Verification items for the finished model (mm, model axes). A direction names the side the tool comes from. Coordinates: 2 decimals unless noted, no trailing zeros. Loops run counter-clockwise (first coordinate to the right, second up) from the corner with the lowest first, then second, coordinate; pieces in that order, holes last.
Q1. Access from +Z, -Z, +X, -X, +Y, -Y to the whole of each face (thin tool, end or side, straight path). Record for faces 4 (the face through (12, 30, -25)), 5 (the face through (82, 42.5, -25)), 6 (the face through (50, 10, -25)), 7 (the face through (11.198, 17.325, -34.915)).
Q2. Sectioned sample at D-D (z = -25). Enter the section's corners in (x, y).
Q3. Sectioned sample at A-A (x = 12.5). Enter the section's corners in (y, z), then the cut area to 3 significant figures.
Q4. Sectioned sample at B-B (y = 6). Enter the section's corners in (x, z), then the cut area to 3 significant figures.
Q5. Go/stop test with flat-tipped pins: P1, Ø1.5, axis at y = 23.5, z = -19.5, coming from the -X side; P2, Ø6, axis at y = 27.5, z = -30.5, coming from the -X side; P3, Ø1.5, axis at x = 10, y = 23, coming from the -Z side. Record where each tip stops, or that it passes through.
Q6. Sectioned sample at C-C (y = 17.5). Enter the section's corners in (x, z).
Q7. Material ranges on probe 1 along X at (y, z) = (6, -21.5); probe 2 along Y at (x, z) = (19.5, -21); probe 3 along Y at (x, z) = (29.5, -5), recorded low to high.
Q8. Mould release check, pull along X, two halves, no side actions. Record for faces 1 (the face through (100, 2, -25)), 2 (the face through (49, 2, -50)), 3 (the face through (38, 5, -25)): +X half, -X half, draft (parallel to the pull), parting line (faces both ways), or undercut.
```python
from build123d import *

# Parameters (mm, degrees)
SKETCH1_W           = 100
SKETCH1_H           = 50
BOSS_EXTRUDE1_DEPTH = 5
SKETCH3_R           = 10
BOSS_EXTRUDE2_DEPTH = 25
SKETCH4_R           = 11.25
BOSS_EXTRUDE3_DEPTH = 5
SKETCH5_R           = 12.5
BOSS_EXTRUDE4_DEPTH = 37.5


with BuildPart() as part:
    # Sketch1 → Boss-Extrude1 (new body)
    with BuildSketch(Plane(origin=(0, 0, 0), x_dir=(1, 0, 0), z_dir=(0, 1, 0))):
        with Locations((50, 25)):
            Rectangle(SKETCH1_W, SKETCH1_H)
    extrude(amount=BOSS_EXTRUDE1_DEPTH)

    # Sketch3 → Boss-Extrude2 (add)
    with BuildSketch(Plane(origin=(0, 5, 0), x_dir=(1, 0, 0), z_dir=(0, 1, 0))):
        with Locations((12.5, 25)):
            Circle(SKETCH3_R)
    extrude(amount=BOSS_EXTRUDE2_DEPTH)

    # Sketch4 → Boss-Extrude3 (add)
    with BuildSketch(Plane(origin=(0, 5, 0), x_dir=(1, 0, 0), z_dir=(0, 1, 0))):
        with Locations((50, 25)):
            Circle(SKETCH4_R)
    extrude(amount=BOSS_EXTRUDE3_DEPTH)

    # Sketch5 → Boss-Extrude4 (add)
    with BuildSketch(Plane(origin=(0, 5, 0), x_dir=(1, 0, 0), z_dir=(0, 1, 0))):
        with Locations((82.5, 25)):
            Circle(SKETCH5_R)
    extrude(amount=BOSS_EXTRUDE4_DEPTH)


solid = part.part
```
Geometry check:
1. face 4: +Z, -Z, -X, +Y
1. face 5: +Z, -Z, +X, -X, +Y
1. face 6: +Z, -Z, +Y
1. face 7: +Y
2. outline: (0, 0) - (100, 0) - (100, 5) - (95, 5) - (95, 42.5) - (70, 42.5) - (70, 5) - (61.25, 5) - (61.25, 10) - (38.75, 10) - (38.75, 5) - (22.5, 5) - (22.5, 30) - (2.5, 30) - (2.5, 5) - (0, 5) - close
3. outline: (0, -50) - (5, -50) - (5, -35) - (30, -35) - (30, -15) - (5, -15) - (5, 0) - (0, 0) - close
3. area: 750 mm2
4. outline: circle Ø20 at (12.5, -25); circle Ø22.5 at (50, -25); circle Ø25 at (82.5, -25)
4. area: 1,200 mm2
5. P1: stops at x = 3.7
5. P2: stops at x = 2.82
5. P3: stops at z = -34.85
6. outline: circle Ø20 at (12.5, -25); circle Ø25 at (82.5, -25)
7. probe 1: x = 3.13 to 21.87, 39.31 to 60.69, 70.5 to 94.5
7. probe 2: y = 0 to 30
7. probe 3: y = 0 to 5
8. face 1: +X half
8. face 2: draft
8. face 3: undercut
